from build123d import *

# Parameters (mm, degrees)
FILLET1_SIZE = 1.5


# Read off the part's stored shape, not the designer's step: Shell1
with BuildPart() as part:
    # Sketch1 → Revolve1 (revolve)
    with BuildSketch(Plane.XY, mode=Mode.PRIVATE) as revolve1_sk:
        Polygon((20, 0), (20, 56.727116956), (21.5, 59.325193167), (21.5, 64.325193167), (19.547262907, 69.998535907), (0, 69.998535907), (0, 2.4), (4.5, 2.4), (4.5, 1.15), (19, 1.15), (19, 0), align=None)
    revolve(revolve1_sk.sketch.rotate(Axis((0, 2.4, 0), (0, 1, 0)), 90), axis=Axis((0, 2.4, 0), (0, 1, 0)))

    # Fillet1
    # the kernel refuses this chamfer: 1.5 mm, written as the material it takes off along each edge
    with BuildSketch(Plane(origin=(0, 1.15, 0), x_dir=(0, 0, -1), z_dir=(1, 0, 0))) as fillet1_piece_1_section:
        Polygon((4.5, FILLET1_SIZE), (4.5 + FILLET1_SIZE, 0), (4.5, 0), align=None)
    fillet1_piece_1 = revolve(axis=Axis((0, 1.15, 0), (0, 1, 0)), mode=Mode.PRIVATE)
    fillet1_piece_1 = split(fillet1_piece_1, bisect_by=Plane(origin=(0, 2.4, 5.37255081), z_dir=(0, -1, 0)), keep=Keep.TOP, mode=Mode.PRIVATE)
    add(fillet1_piece_1, mode=Mode.SUBTRACT)

    # Shell1 outline → Shell1 (revolve, cut)
    with BuildSketch(Plane.XY):
        Polygon((18.489685342, 69.998535907), (0, 69.998535907), (0, 3.4), (5.164213562, 3.4), (6.414213562, 2.15), (19, 2.15), (19, 56.995066148), (20.5, 59.59314236), (20.5, 64.157911426), align=None)
    revolve(axis=Axis((0, 0, 0), (0, 1, 0)), mode=Mode.SUBTRACT)


solid = part.part
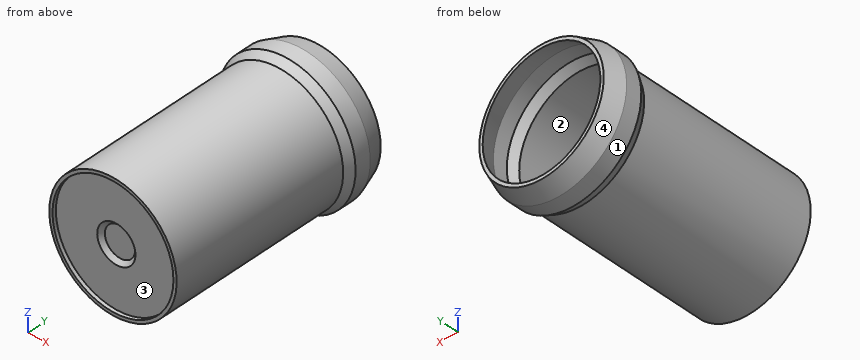
Geometry: final body of the model. Coordinates: model frame, mm. Face numbers are marked on the shaded views. A direction names the side the tool comes from. Give positions to 0.01 mm unless a question says otherwise; leave off trailing zeros. Loops run counter-clockwise (first coordinate to the right, second up) from the corner with the lowest first, then second, coordinate; pieces in that order, holes last. Notation, with made-up numbers: M -9.75,-38 L 1.25,-38 A33 ccw 1.25,-4 Z; hole C 86,32.25 d9. An arc over 180 degrees is marked long. Put each result on its own line as item: value.
1) Reachability of the marked faces 3 and 4 from +Z, -Z, +X, -X, +Y, -Y: full face, straight path, thin tool, end or side. Return the list, or none.
Computed values:
face 3: -Y
face 4: +Y
2) Mould query, pull axis Z, two halves, no side actions, for the marked faces 1 and 2. Classes: released by +Z, released by -Z, zero draft, split by the parting line, or undercut.
Computed values:
face 1: split by the parting line
face 2: undercut
3) Cut plane A-A, the plane y = 37. Return the cut outline in (x, z).
Computed values:
outline: C 0,0 d40; hole C 0,0 d38
4) First-contact query: P1, Ø3, axis at x = -1, z = -1, coming from the -Y side; P2, Ø3, axis at x = -6, y = 31.5, coming from the -Z side; P3, Ø8, axis at x = 11, y = 62, coming from the -Z side; P4, Ø3, axis at x = -17, z = 9, coming from the -Y side. Flat tips, straight axial feed; report the tip coordinate or a pass-through.
Computed values:
P1: stops at y = 2.4
P2: stops at z = -19.49
P3: stops at z = -20.33
P4: stops at y = 0
5) Material intervals for L1, parallel to X at y = 25.5, z = 0; L2, parallel to Z at x = -0.5, y = 27; L3, parallel to X at y = 61.4, z = 0, sorted ascending. Write a range as from..to.
Computed values:
L1: x = -20..-19, 19..20
L2: z = -19.99..-18.99, 18.99..19.99
L3: x = -21.5..-20.5, 20.5..21.5
